CAD build for the part. Positions are in the model's coordinates, mm. A direction names the side the tool comes from. Coordinates: 2 decimals unless noted, no trailing zeros. Loops run counter-clockwise (first coordinate to the right, second up) from the corner with the lowest first, then second, coordinate; pieces in that order, holes last. Notation, with made-up numbers: (47, 29.5) - (81, 29.5) arc R15 ccw to (81, 51.5) - close; hole circle Ø4 at (-30.5, 1.5). An arc over 180 degrees is marked (long way). Put each result on its own line as item: value.
```python
from build123d import *

# Parameters (mm, degrees)
MOTOR_BASE_R                    = 35
STATOR_SHELL_DEPTH              = 65
MOTOR_BASE_4_R                  = 18.75
MOTOR_BASE_4_R_2                = 4.7625
MOTOR_BASE_4_R_3                = 3.175
CUT_EXTRUDE1_DEPTH              = 82.700673192
STATOR_LAMINATION_SUPPORT_DEPTH = 16.35
CUT_EXTRUDE3_DEPTH              = 82.700673192


with BuildPart() as part:
    # Motor_Base → Stator_Shell (new body)
    with BuildSketch(Plane.XY):
        Circle(MOTOR_BASE_R)
        with BuildLine():
            Line((1.533091596, 21.069409042), (1.533091596, 33.069409042))
            ThreePointArc((1.533091596, 33.069409042), (16.733091596, 28.996581317), (27.860263871, 17.869409042))
            Line((27.860263871, 17.869409042), (17.467959025, 11.869409042))
            Line((17.467959025, 11.869409042), (1.533091596, 21.069409042))
        make_face(mode=Mode.SUBTRACT)
        with BuildLine():
            Line((-1.533091596, 21.069409042), (-1.533091596, 33.069409042))
            ThreePointArc((-1.533091596, 33.069409042), (-16.733091596, 28.996581317), (-27.860263871, 17.869409042))
            Line((-27.860263871, 17.869409042), (-17.467959025, 11.869409042))
            Line((-17.467959025, 11.869409042), (-1.533091596, 21.069409042))
        make_face(mode=Mode.SUBTRACT)
        with BuildLine():
            Line((19.001050621, 9.214016506), (29.393355467, 15.214016506))
            ThreePointArc((29.393355467, 15.214016506), (33.466183191, 0.014016506), (29.393355467, -15.185983494))
            Line((29.393355467, -15.185983494), (19.001050621, -9.185983494))
            Line((19.001050621, -9.185983494), (19.001050621, 9.214016506))
        make_face(mode=Mode.SUBTRACT)
        with BuildLine():
            Line((17.467959025, -11.841376031), (27.860263871, -17.841376031))
            ThreePointArc((27.860263871, -17.841376031), (16.733091596, -28.968548306), (1.533091596, -33.041376031))
            Line((1.533091596, -33.041376031), (1.533091596, -21.041376031))
            Line((1.533091596, -21.041376031), (17.467959025, -11.841376031))
        make_face(mode=Mode.SUBTRACT)
        with BuildLine():
            Line((-1.533091596, -21.041376031), (-1.533091596, -33.041376031))
            ThreePointArc((-1.533091596, -33.041376031), (-16.733091596, -28.968548306), (-27.860263871, -17.841376031))
            Line((-27.860263871, -17.841376031), (-17.467959025, -11.841376031))
            Line((-17.467959025, -11.841376031), (-1.533091596, -21.041376031))
        make_face(mode=Mode.SUBTRACT)
        with BuildLine():
            Line((-19.001050621, -9.185983494), (-29.393355467, -15.185983494))
            ThreePointArc((-29.393355467, -15.185983494), (-33.466183191, 0.014016506), (-29.393355467, 15.214016506))
            Line((-29.393355467, 15.214016506), (-19.001050621, 9.214016506))
            Line((-19.001050621, 9.214016506), (-19.001050621, -9.185983494))
        make_face(mode=Mode.SUBTRACT)
    extrude(amount=STATOR_SHELL_DEPTH)

    # Motor_Base_4 → Cut-Extrude1 (cut, through all)
    # profile 1 of 3: a face of its own
    with BuildSketch(Plane.XY):
        Circle(MOTOR_BASE_4_R)
        Circle(MOTOR_BASE_4_R_2, mode=Mode.SUBTRACT)
    # profile 2 of 3: a face of its own
    with BuildSketch(Plane.XY):
        Circle(MOTOR_BASE_4_R_2)
        Circle(MOTOR_BASE_4_R_3, mode=Mode.SUBTRACT)
    # profile 3 of 3: a face of its own
    with BuildSketch(Plane.XY):
        Circle(MOTOR_BASE_4_R_3)
    extrude(amount=CUT_EXTRUDE1_DEPTH, mode=Mode.SUBTRACT)

    # Stator_Lam_Support → Stator Lamination Support (add)
    with BuildSketch(Plane(origin=(0, 0, 0), x_dir=(-1, 0, 0), z_dir=(0, 0, -1))):
        with BuildLine():
            Line((14.351295245, 31.306334292), (13.506552589, 28.096442893))
            Line((13.506552589, 28.096442893), (17.559972866, 25.758191299))
            Line((17.559972866, 25.758191299), (19.915725917, 28.096442893))
            ThreePointArc((19.915725917, 28.096442893), (17.208516366, 29.831413083), (14.351295245, 31.306334292))
        make_face()
        with BuildLine():
            Line((34.287728419, 3.224580887), (31.085509595, 2.351203787))
            Line((31.085509595, 2.351203787), (31.087234454, -2.328286942))
            Line((31.087234454, -2.328286942), (34.29009626, -3.199303133))
            ThreePointArc((34.29009626, -3.199303133), (34.439019743, 0.012694207), (34.287728419, 3.224580887))
        make_face()
        with BuildLine():
            Line((19.936433174, -28.081753405), (17.578957007, -25.745239106))
            Line((17.578957007, -25.745239106), (13.527261587, -28.086478241))
            Line((13.527261587, -28.086478241), (14.374370343, -31.295746025))
            ThreePointArc((14.374370343, -31.295746025), (17.230503377, -29.818718876), (19.936433174, -28.081753405))
        make_face()
        with BuildLine():
            Line((-14.351295245, -31.306334292), (-13.506552589, -28.096442893))
            Line((-13.506552589, -28.096442893), (-17.559972866, -25.758191299))
            Line((-17.559972866, -25.758191299), (-19.915725917, -28.096442893))
            ThreePointArc((-19.915725917, -28.096442893), (-17.208516366, -29.831413083), (-14.351295245, -31.306334292))
        make_face()
        with BuildLine():
            Line((-34.287728419, -3.224580887), (-31.085509595, -2.351203787))
            Line((-31.085509595, -2.351203787), (-31.087234454, 2.328286942))
            Line((-31.087234454, 2.328286942), (-34.29009626, 3.199303133))
            ThreePointArc((-34.29009626, 3.199303133), (-34.439019743, -0.012694207), (-34.287728419, -3.224580887))
        make_face()
        with BuildLine():
            Line((-19.936433174, 28.081753405), (-17.578957007, 25.745239106))
            Line((-17.578957007, 25.745239106), (-13.527261587, 28.086478241))
            Line((-13.527261587, 28.086478241), (-14.374370343, 31.295746025))
            ThreePointArc((-14.374370343, 31.295746025), (-17.230503377, 29.818718876), (-19.936433174, 28.081753405))
        make_face()
    extrude(amount=-STATOR_LAMINATION_SUPPORT_DEPTH)

    # Sketch6 → Cut-Extrude3 (cut, through all)
    with BuildSketch(Plane.XY.offset(65)):
        Polygon((14.405256844, 16.666586459), (11.56399771, 11.741189457), (4.374457659, 15.888539677), (7.215716793, 20.813936679), align=None)
        Polygon((21.633256314, 4.15797429), (21.63631569, -4.142025146), (15.950167195, -4.144121058), (15.947107819, 4.155878379), align=None)
        Polygon((14.417539521, -16.655962389), (7.231058845, -20.808611605), (4.386169485, -15.885310514), (11.57265016, -11.732661299), align=None)
        Polygon((-7.215716793, -20.813936679), (-14.405256844, -16.666586459), (-11.56399771, -11.741189457), (-4.374457659, -15.888539677), align=None)
        Polygon((-21.633256314, -4.15797429), (-21.63631569, 4.142025146), (-15.950167195, 4.144121058), (-15.947107819, -4.155878379), align=None)
        Polygon((-14.417539521, 16.655962389), (-7.231058845, 20.808611605), (-4.386169485, 15.885310514), (-11.57265016, 11.732661299), align=None)
    extrude(amount=-CUT_EXTRUDE3_DEPTH, mode=Mode.SUBTRACT)


solid = part.part
```
Q1. Slice it at B-B, the plane y = 0. Give the cut face in (x, z), then the cut area to 3 significant figures.
Determined:
outline: (-35, 0) - (-31.09, 0) - (-31.09, 16.35) - (-33.47, 16.35) - (-33.47, 65) - (-35, 65) - close; (31.09, 0) - (35, 0) - (35, 65) - (33.47, 65) - (33.47, 16.35) - (31.09, 16.35) - close
area: 277 mm2
Q2. Pin check, flat tips, straight feed: pin 1 Ø4 at (y, z) = (-7.5, 46.5) entering from +X; pin 2 Ø4 at (y, z) = (6.5, 25) entering from +X; pin 3 Ø6 at (y, z) = (24.5, 17) entering from -X. Stop position of each tip, or through.
Determined:
pin 1: x = 34.57
pin 2: x = 34.71
pin 3: x = -27.62
Q3. Tool access for faces 1 (the flat face through (1.533, -27, 32)), 2 (the flat face through (-16, -28, 16.35)): list every direction of +Z, -Z, +X, -X, +Y, -Y with a clear straight run to the whole face (end or side of a thin tool).
Determined:
face 1: +Z, -Z
face 2: +Z
Q4. Slice it at A-A, the plane x = 0. Give the cut face in (y, z), then the cut area to 3 significant figures.
Determined:
outline: (-35, 0) - (-18.75, 0) - (-18.75, 65) - (-35, 65) - close; (18.75, 0) - (35, 0) - (35, 65) - (18.75, 65) - close
area: 2,110 mm2
Q5. Slice it at D-D, the plane y = -23. Give the cut face in (x, z).
Determined:
outline: (-26.38, 0) - (-24.11, 0) - (-24.11, 65) - (-26.38, 65) - close; (-1.53, 0) - (1.53, 0) - (1.53, 65) - (-1.53, 65) - close; (24.11, 0) - (26.38, 0) - (26.38, 65) - (24.11, 65) - close
Q6. Mould opens along Y. For faces 3 (the cylindrical face through (-28, -21, 32)), 4 (the flat face through (-18.3, -5, 65)), 5 (the flat face through (32.19, 2.63, 8.06)) say: +Y half, -Y half, draft (parallel to the pull), parting line (faces both ways), or undercut.
Determined:
face 3: parting line
face 4: draft
face 5: undercut
Q7. Slice it at C-C, the plane x = 24.5. Give the cut face in (y, z) (3 decimals).
Determined:
outline: (-24.995, 0) - (-22.558, 0) - (-22.558, 65) - (-24.995, 65) - close; (-15.901, 0) - (-12.361, 0) - (-12.361, 65) - (-15.901, 65) - close; (12.389, 0) - (15.929, 0) - (15.929, 65) - (12.389, 65) - close; (22.586, 0) - (24.995, 0) - (24.995, 65) - (22.586, 65) - close
Q8. Wall check: L1, parallel to Y at x = 17, z = 25; L2, parallel to Y at x = -20.5, z = 20.5; L3, parallel to X at y = -7, z = 14.5. Give the ranges that are in metal, low to high. Write a range as from..to.
Determined:
L1: -30.59..-28.81, -12.11..-7.91, 7.91..12.14, 28.84..30.59
L2: -28.37..-26.4, -13.59..-10.05, 10.08..13.62, 26.43..28.37
L3: -34.29..-32.65, -19..-17.39, 17.39..19, 32.65..34.29
